```python
from build123d import *

# Parameters (mm, degrees)
SKETCH2_R           = 10
BOSS_EXTRUDE1_DEPTH = 15


with BuildPart() as part:
    # Sketch1 → Revolve1 (revolve)
    with BuildSketch(Plane.XY, mode=Mode.PRIVATE) as revolve1_sk:
        Polygon((0, 0), (40, 0), (40, -90), (30, -90), (30, -10), (0, -10), align=None)
    revolve(revolve1_sk.sketch.rotate(Axis((0, -10, 0), (0, -1, 0)), 180), axis=Axis((0, -10, 0), (0, -1, 0)))

    # Sketch2 → Boss-Extrude1 (add, symmetric)
    with BuildSketch(Plane(origin=(0, 0, 0), x_dir=(0, 0, -1), z_dir=(1, 0, 0))):
        with BuildLine():
            Line((-25, 30), (-25, 0))
            Line((-25, 0), (25, 0))
            Line((25, 0), (25, 30))
            ThreePointArc((25, 30), (0, 55), (-25, 30))
        make_face()
        with Locations((0, 30)):
            Circle(SKETCH2_R, mode=Mode.SUBTRACT)
    extrude(amount=BOSS_EXTRUDE1_DEPTH, both=True)


solid = part.part
```
The model under review builds one solid part; all positions refer to its coordinate system, in mm. A direction names the side the tool comes from. Coordinates: 2 decimals unless noted, no trailing zeros. Order: outer loops, then holes, each group sorted by start corner. A loop starts at its lowest first (then second) coordinate and runs counter-clockwise, first axis right, second up. Notation, with made-up numbers: (77, 68.25) -> (134, 68.25) arc R20 ccw to (134, 79.25) -> close; hole circle Ø8 at (9.5, 47). An arc over 180 degrees is marked (long way). Answer in a Markdown table with one row per item. Add a question column.
Item 1: We need section D-D on y = -63. Write out the cut boundary in (x, z), plus the area to 3 significant figures.
Item 2: Clearance check with flat-ended pins moving along their axes: pin 1 (10 mm diameter, centred on x = 24.5, z = 10, fed in from -Y); pin 2 (2 mm diameter, centred on x = -20, z = -23, fed in from +Y); pin 3 (15 mm diameter, centred on x = 4, y = 14.5, fed in from -Z); pin 4 (8 mm diameter, centred on y = -31, z = 5, fed in from -X). State where each tip first meets the part, or that it passes through.
Item 3: Mouldability with a two-part tool opening along X and no side actions: class faces 6 (the flat face through (0, 15, 25)), 7 (the flat face through (0, -10, 0)), 8 (the flat face through (-15, 16, 0)) as +X half, -X half, draft (parallel to the pull), parting line (faces both ways), or undercut.
Item 4: To check wall thickness, follow probe 1 along Z at (x, y) = (0, -46.5); probe 2 along Y at (x, z) = (-8, 0); probe 3 along Z at (x, y) = (-25, -78.5). State the ranges of each line that lie inside material, in increasing order.
Item 5: We need section B-B on x = 0. Write out the cut boundary in (y, z), plus the area to 3 significant figures.
Item 6: We need section C-C on x = -23. Write out the cut boundary in (y, z), plus the area to 3 significant figures.
Item 7: Machinability: for faces 1 (the cylindrical face through (-16.128, -49.44, -25.296)), 2 (the flat face through (15, 16, 0)), 3 (the cylindrical face through (-0.21, 20.24, 2.17)), 4 (the flat face through (-6, -90, -30)), 5 (the flat face through (0, 15, -25)), which of the approach directions +Z, -Z, +X, -X, +Y, -Y give a long, thin tool a straight path to every point of the face, cutting with its end or side? Answer none if there is none.
Item 8: We need section A-A on z = 0. Write out the cut boundary in (x, y).
Final values:
| question | item | result |
|---|---|---|
| 1 | outline | circle Ø80 at (0, 0); hole circle Ø60 at (0, 0) |
| 1 | area | 2,200 mm2 |
| 2 | pin 1 | stops at y = -90 |
| 2 | pin 2 | stops at y = 0 |
| 2 | pin 3 | stops at z = -25 |
| 2 | pin 4 | stops at x = -39.99 |
| 3 | face 6 | draft |
| 3 | face 7 | undercut |
| 3 | face 8 | -X half |
| 4 | probe 1 | z = -40 to -30, 30 to 40 |
| 4 | probe 2 | y = -10 to 20, 40 to 55 |
| 4 | probe 3 | z = -31.22 to -16.58, 16.58 to 31.22 |
| 5 | outline | (-90, -40) -> (0, -40) -> (0, -25) -> (30, -25) arc R25 ccw to (30, 25) -> (0, 25) -> (0, 40) -> (-90, 40) -> (-90, 30) -> (-10, 30) -> (-10, -30) -> (-90, -30) -> close; hole circle Ø20 at (30, 0) |
| 5 | area | 4,570 mm2 |
| 6 | outline | (-90, -32.73) -> (0, -32.73) -> (0, 32.73) -> (-90, 32.73) -> (-90, 19.26) -> (-10, 19.26) -> (-10, -19.26) -> (-90, -19.26) -> close |
| 6 | area | 2,810 mm2 |
| 7 | face 1 | -Y |
| 7 | face 2 | +Z, -Z, +X, +Y |
| 7 | face 3 | +X, -X |
| 7 | face 4 | +Z, -Z, +X, -X, -Y |
| 7 | face 5 | -Z, +X, -X, +Y |
| 8 | outline | (-40, -90) -> (-30, -90) -> (-30, -10) -> (30, -10) -> (30, -90) -> (40, -90) -> (40, 0) -> (15, 0) -> (15, 20) -> (-15, 20) -> (-15, 0) -> (-40, 0) -> close; (-15, 40) -> (15, 40) -> (15, 55) -> (-15, 55) -> close |
